from build123d import *

# Parameters (mm, degrees)
SKETCH020_W     = 5
SKETCH020_H     = 21.2
PAD010_DEPTH    = 9
SKETCH023_W     = 6.65
SKETCH023_H     = 8.1
POCKET011_DEPTH = 4
SKETCH024_R     = 1.05
POCKET012_DEPTH = 10
SKETCH025_R     = 2
POCKET013_DEPTH = 3


with BuildPart() as part:
    # Sketch020 → Pad010 (new body)
    with BuildSketch(Plane.XZ):
        with Locations((26.859407, 7.981561)):
            Rectangle(SKETCH020_W, SKETCH020_H)
    extrude(amount=PAD010_DEPTH)

    # Sketch023 (on Face5 of Pad010) → Pocket011 (cut)
    with BuildSketch(Plane(origin=(0, 0, 0), x_dir=(1, 0, 0), z_dir=(0, 1, 0))):
        with Locations((27.211889, -8.03451)):
            Rectangle(SKETCH023_W, SKETCH023_H)
    extrude(amount=-POCKET011_DEPTH, mode=Mode.SUBTRACT)

    # Sketch024 (on Face2 of Pocket011) → Pocket012 (cut)
    with BuildSketch(Plane(origin=(0, 0, 0), x_dir=(1, 0, 0), z_dir=(0, 1, 0))):
        with Locations((27.009228, -13.650866)):
            Circle(SKETCH024_R)
        with Locations((27.036736, -2.243972)):
            Circle(SKETCH024_R)
    extrude(amount=-POCKET012_DEPTH, mode=Mode.SUBTRACT)

    # Sketch025 (on Face8 of Pocket012) → Pocket013 (cut)
    with BuildSketch(Plane.XZ.offset(9)):
        with Locations((27.009228, 13.650866)):
            Circle(SKETCH025_R)
        with Locations((27.036736, 2.243972)):
            Circle(SKETCH025_R)
    extrude(amount=-POCKET013_DEPTH, mode=Mode.SUBTRACT)


with BuildPart() as part_1:
    # Body005 placement: moved
    add(part.part.moved(Location((0, 20, 0))))


solid = part_1.part
Work out the finished part from the listing and answer in its coordinate system (mm). A direction names the side the tool comes from. Give positions to 0.01 mm unless a question says otherwise; leave off trailing zeros. Write each loop counter-clockwise with the first axis right and the second up, starting at its lowest first coordinate (ties: lowest second). Pieces come first, ordered by that corner, then holes.
Q1. The part is cut by section C-C on x = 26.4. Give the vertices of the cut face in (y, z).
Answer:
outline: (11, -2.62) - (20, -2.62) - (20, 1.41) - (14, 1.41) - (14, 0.35) - (11, 0.35) - close; (11, 4.14) - (14, 4.14) - (14, 3.08) - (20, 3.08) - (20, 3.98) - (16, 3.98) - (16, 12.08) - (20, 12.08) - (20, 12.8) - (14, 12.8) - (14, 11.75) - (11, 11.75) - close; (11, 15.56) - (14, 15.56) - (14, 14.51) - (20, 14.51) - (20, 18.58) - (11, 18.58) - close
Q2. The part is cut by section B-B on z = 3. Give the vertices of the cut face in (x, y), and give its area (3 significant figures).
Answer:
outline: (24.36, 11) - (25.19, 11) - (25.19, 14) - (26.31, 14) - (26.31, 20) - (24.36, 20) - close; (27.77, 14) - (28.89, 14) - (28.89, 11) - (29.36, 11) - (29.36, 20) - (27.77, 20) - close
area: 25.1 mm2
Q3. The part is cut by section A-A on y = 19.25. Give the vertices of the cut face in (x, z), and give its area (3 significant figures).
Answer:
outline: (24.36, -2.62) - (29.36, -2.62) - (29.36, 3.98) - (24.36, 3.98) - close; (24.36, 12.08) - (29.36, 12.08) - (29.36, 18.58) - (24.36, 18.58) - close; hole circle Ø2.1 at (27.01, 13.65); hole circle Ø2.1 at (27.04, 2.24)
area: 58.6 mm2
Q4. Straight lines are drawn through the part: L1, parallel to Z at x = 28.2, y = 12.75; L2, parallel to Z at x = 25.4, y = 13.25; L3, parallel to Z at x = 29, y = 18. For each, find the intervals that lie inside material, in ascending order.
Answer:
L1: z = -2.62 to 0.62, 3.87 to 12.04, 15.26 to 18.58
L2: z = -2.62 to 1.09, 3.39 to 12.46, 14.84 to 18.58
L3: z = -2.62 to 3.98, 12.08 to 18.58
Q5. Given pin 1 (1.5 mm diameter, centred on x = 26, z = 6.5, fed in from +Y); pin 2 (1.2 mm diameter, centred on x = 27, z = 14.5, fed in from -Y), each flat-ended and moving along its own axis, determine where each tip first touches the part or whether it passes through.
Answer:
pin 1: stops at y = 16
pin 2: stops at y = 14
Q6. For a pull along Z with two mould halves and no side action, classify faces 1 (the face through (27, 16, 8)), 2 (the face through (28, 14, 1)), 3 (the face through (27, 20, 1)), 4 (the face through (27, 16, -2.618)) as released by +Z, released by -Z, zero draft, split by the parting line, or undercut.
Answer:
face 1: undercut
face 2: undercut
face 3: zero draft
face 4: released by -Z
Q7. A tool of negligible diameter and unlimited length cuts with its end or side. For faces 5 (the face through (28.04, 17.04, 1.93)), 6 (the face through (27.9, 14, 12.8)), 7 (the face through (27, 18, 3.985)), from which of +Z, -Z, +X, -X, +Y, -Y can it reach the whole face along a straight path? Write none if from no direction.
Answer:
face 5: +Y, -Y
face 6: -Y
face 7: +X, -X, +Y
Q8. The part is cut by section D-D on x = 28.45. Give the vertices of the cut face in (y, z), and give its area (3 significant figures).
Answer:
outline: (11, -2.62) - (20, -2.62) - (20, 3.98) - (16, 3.98) - (16, 12.08) - (20, 12.08) - (20, 18.58) - (11, 18.58) - (11, 15.04) - (14, 15.04) - (14, 12.26) - (11, 12.26) - (11, 3.66) - (14, 3.66) - (14, 0.83) - (11, 0.83) - close
area: 142 mm2
